For this review, take the finished solid that the model builds, in its own axes (mm). A direction names the side the tool comes from. Coordinates: 2 decimals unless noted, no trailing zeros. Order: outer loops, then holes, each group sorted by start corner. A loop starts at its lowest first (then second) coordinate and runs counter-clockwise, first axis right, second up. Notation, with made-up numbers: (66, -14) - (116, -14) arc R9 ccw to (116, 0) - close; hole circle Ø3 at (61.25, 57). An arc over 180 degrees is marked (long way). One line per item, written item: value. Start each with the question number.
(1) Consider section C-C on y = 3.5. Write out the cut boundary in (x, z).
(2) Consider section B-B on x = -19.5. Write out the cut boundary in (y, z).
(3) To check wall thickness, follow line 1 along Z through (x, y) = (-18.25, 17.5); line 2 along X through (y, z) = (12.75, -6.75); line 3 along X through (y, z) = (3, -5.25). State the ranges of each line that lie inside material, in increasing order.
(4) Consider section D-D on x = -12.5. Write out the cut boundary in (y, z).
(5) Mouldability with a two-part tool opening along X and no side actions: class faces 1 (the flat face through (-15, 19.05, -4)), 2 (the cylindrical face through (-18.07, 9.39, -1.78)), 3 (the flat face through (-18.43, 10, -9)), 4 (the cylindrical face through (-18.45, 9.39, 2.11)) as released by +X, released by -X, zero draft, split by the parting line, or undercut.
(6) Consider section A-A on z = -9.5. Write out the cut boundary in (x, y), then the cut area to 3 significant figures.
(7) For faces 5 (the flat face through (-17.922, 10, -9)), 6 (the flat face through (-15, 0, -4)), list the 3-axis set-ups (+Z, -Z, +X, -X, +Y, -Y) from which the entire face can be reached by the end or side of a thin tool; tool diameter is ignored.
(8) Clearance check with flat-ended pins moving along their axes: pin 1 (1 mm diameter, centred on x = -14.5, y = 15.5, fed in from +Z); pin 2 (1.2 mm diameter, centred on y = 12, z = -8, fed in from -X); pin 3 (2 mm diameter, centred on y = 6, z = -1.5, fed in from +X); pin 4 (3 mm diameter, centred on x = -18.18, z = -4.23, fed in from +Y). State where each tip first meets the part, or that it passes through.
```python
from build123d import *

# Parameters (mm, degrees)
SKETCH1_R                    = 6.35
BOSS_EXTRUDE1_DEPTH          = 19.05
F_10_0_1935_DIAMETER_HOLE2_D = 4.9149
CUT_EXTRUDE1_DEPTH           = 33.808987893


with BuildPart() as part:
    # Sketch1 → Boss-Extrude1 (new body)
    with BuildSketch(Plane(origin=(0, 0, 0), x_dir=(1, 0, 0), z_dir=(0, 1, 0))):
        with Locations(Location((-18.175558327, 4.234147358, 0), (0, 0, 90))):
            Circle(SKETCH1_R)
    extrude(amount=BOSS_EXTRUDE1_DEPTH)

    # #10 (0.1935) Diameter Hole2 (through all)
    with Locations(Plane(origin=(0, 19.05, 0), x_dir=(1, 0, 0), z_dir=(0, 1, 0))):
        with Locations((-18.175558327, 4.234147358)):
            Hole(F_10_0_1935_DIAMETER_HOLE2_D / 2)

    # Sketch6 → Cut-Extrude1 (cut, through all)
    with BuildSketch(Plane(origin=(0, 19.05, 0), x_dir=(1, 0, 0), z_dir=(0, 1, 0))):
        with BuildLine():
            Line((-18.429558327, 10.579065324), (-18.429558327, 6.678435496))
            ThreePointArc((-18.429558327, 6.678435496), (-18.175558327, 6.691597358), (-17.921558327, 6.678435496))
            Line((-17.921558327, 6.678435496), (-17.921558327, 10.579065324))
            ThreePointArc((-17.921558327, 10.579065324), (-18.175558327, 10.584147358), (-18.429558327, 10.579065324))
        make_face()
    extrude(amount=-CUT_EXTRUDE1_DEPTH, mode=Mode.SUBTRACT)


solid = part.part
```
Geometry check:
1. outline: (-18.43, -10.58) - (-18.43, -6.68) arc R2.46 cw (long way) to (-17.92, -6.68) - (-17.92, -10.58) arc R6.35 ccw (long way) to start
2. outline: (0, -10.44) - (19.05, -10.44) - (19.05, -6.3) - (0, -6.3) - close; (0, -2.16) - (19.05, -2.16) - (19.05, 1.98) - (0, 1.98) - close
3. line 1: z = -1.78 to 2.12
3. line 2: x = -24.01 to -18.43, -17.92 to -12.35
3. line 3: x = -24.44 to -20.41, -15.94 to -11.91
4. outline: (0, -7.08) - (19.05, -7.08) - (19.05, -1.39) - (0, -1.39) - close
5. face 1: zero draft
5. face 2: undercut
5. face 3: undercut
5. face 4: split by the parting line
6. outline: (-21.72, 0) - (-18.43, 0) - (-18.43, 19.05) - (-21.72, 19.05) - close; (-17.92, 0) - (-14.63, 0) - (-14.63, 19.05) - (-17.92, 19.05) - close
6. area: 126 mm^2
7. face 5: -Z, +Y, -Y
7. face 6: +Z, -Z, +X, -X, -Y
8. pin 1: stops at z = 1.26
8. pin 2: stops at x = -23.68
8. pin 3: stops at x = -12.07
8. pin 4: passes through
